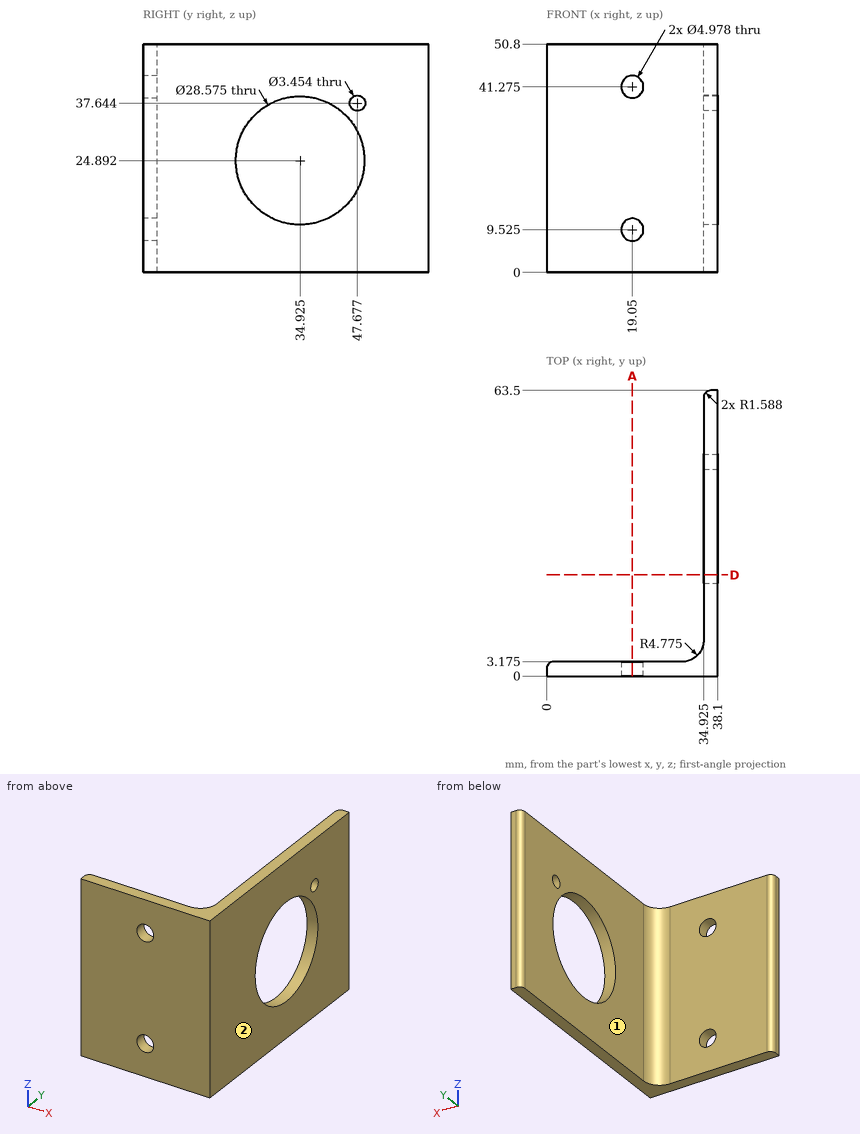
Here's the drawing with two shaded views (mm, measured from the low corner). I have some questions. A direction names the side the tool comes from. Give positions to 0.01 mm unless a question says otherwise; leave off trailing zeros. Write each loop counter-clockwise with the first axis right and the second up, starting at its lowest first coordinate (ties: lowest second). Pieces come first, ordered by that corner, then holes. Notation, with made-up numbers: (71.5, 10) - (123.5, 10) arc R13 cw to (123.5, 34) - close; hole circle Ø9 at (-37.75, -14.5). An arc over 180 degrees is marked (long way). One line per item, written item: value. Start each with the question number.
Item 1: Imagine slicing it at D-D, the plane y = 22.5. List the corners of the cut face in (x, z) for me (1 decimal).
Item 2: I'm going to push flat-ended pins straight in: pin 1 (1.5 mm diameter, centred on x = 23, z = 9.5, fed in from +Y) (1 decimal); pin 2 (12 mm diameter, centred on x = 28.5, y = 52.5, fed in from +Z); pin 3 (5 mm diameter, centred on x = 11, z = 15.5, fed in from -Y); pin 4 (1 mm diameter, centred on y = 20, z = 44.5, fed in from -X) (1 decimal). Where does each tip first touch, or does it pass through?
Item 3: Imagine slicing it at A-A, the plane x = 19.05. List the corners of the cut face in (y, z) for me (1 decimal).
Item 4: Which directions (+Z, -Z, +X, -X, +Y, -Y) give clear straight access to the entire face, cutting with the end or side of a thin tool? Please do the marked faces 1 and 2.
Item 5: Please list where these lines run through material, in increasing order: line 1 (Z direction, x = 19.05, y = 2.45) (1 decimal); line 2 (Y direction, x = 15, z = 22) (1 decimal); line 3 (X direction, y = 53, z = 45) (1 decimal). Write a range as from..to.
Geometry says:
1. outline: (34.9, 0) - (38.1, 0) - (38.1, 17.8) - (34.9, 17.8) - close; (34.9, 31.9) - (38.1, 31.9) - (38.1, 50.8) - (34.9, 50.8) - close
2. pin 1: y = 3.2
2. pin 2: through
2. pin 3: y = 0
2. pin 4: x = 34.9
3. outline: (0, 0) - (3.2, 0) - (3.2, 7) - (0, 7) - close; (0, 12) - (3.2, 12) - (3.2, 38.8) - (0, 38.8) - close; (0, 43.8) - (3.2, 43.8) - (3.2, 50.8) - (0, 50.8) - close
4. face 1: +Z, -Z, -X, +Y
4. face 2: +Z, -Z, +X, +Y, -Y
5. line 1: 0..7, 12..38.8, 43.8..50.8
5. line 2: 0..3.2
5. line 3: 34.9..38.1
